Build history of the part. All positions in model axes, mm. Round coordinates to 2 decimals unless told otherwise and drop trailing zeros. Write each loop counter-clockwise with the first axis right and the second up, starting at its lowest first coordinate (ties: lowest second). Pieces come first, ordered by that corner, then holes.
from build123d import *

# Parameters (mm, degrees)
EXTRUDE_1_DEPTH     = 75
CUT_EXTRUDE_1_DEPTH = 5


with BuildPart() as part:
    # ｽｹｯﾁ1 → ﾎﾞｽ - 押し出し1 (new body)
    with BuildSketch(Plane(origin=(0, 0, 0), x_dir=(1, 0, 0), z_dir=(0, 1, 0))):
        with BuildLine():
            Line((-4, -5), (4, -5))
            ThreePointArc((4, -5), (4.707106781, -4.707106781), (5, -4))
            Line((5, -4), (5, 4))
            ThreePointArc((5, 4), (4.707106781, 4.707106781), (4, 5))
            Line((4, 5), (-4, 5))
            ThreePointArc((-4, 5), (-4.707106781, 4.707106781), (-5, 4))
            Line((-5, 4), (-5, -4))
            ThreePointArc((-5, -4), (-4.707106781, -4.707106781), (-4, -5))
        make_face()
    extrude(amount=EXTRUDE_1_DEPTH)

    # ｽｹｯﾁ2 → ｶｯﾄ - 押し出し1 (cut)
    with BuildSketch(Plane(origin=(0, 75, 0), x_dir=(1, 0, 0), z_dir=(0, 1, 0))):
        with BuildLine():
            Line((-1.6, -2.6), (1.6, -2.6))
            ThreePointArc((1.6, -2.6), (2.307106781, -2.307106781), (2.6, -1.6))
            Line((2.6, -1.6), (2.6, 1.6))
            ThreePointArc((2.6, 1.6), (2.307106781, 2.307106781), (1.6, 2.6))
            Line((1.6, 2.6), (-1.6, 2.6))
            ThreePointArc((-1.6, 2.6), (-2.307106781, 2.307106781), (-2.6, 1.6))
            Line((-2.6, 1.6), (-2.6, -1.6))
            ThreePointArc((-2.6, -1.6), (-2.307106781, -2.307106781), (-1.6, -2.6))
        make_face()
    extrude(amount=-CUT_EXTRUDE_1_DEPTH, mode=Mode.SUBTRACT)


solid = part.part
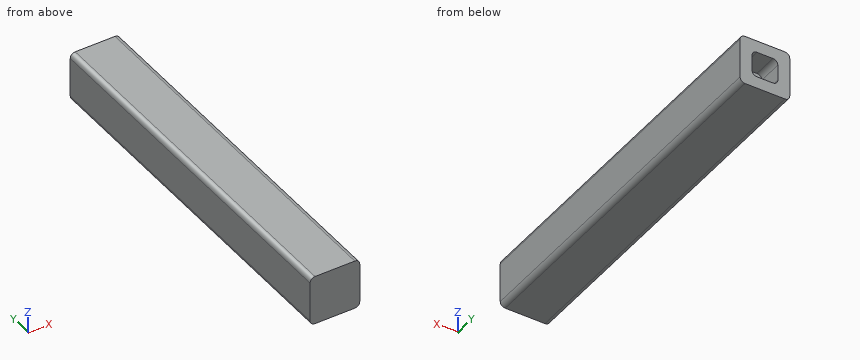
1) Wall check: L1, parallel to Y at x = 2.25, z = -0.5; L2, parallel to X at y = 43.5, z = -4.25; L3, parallel to X at y = 63, z = 4.5. Give the ranges that are in metal, low to high.
Results:
L1: y = 0 to 70
L2: x = -4.97 to 4.97
L3: x = -4.87 to 4.87
2) Slice it at A-A (x = -0.25). Write the cut outline in (y, z), plus the area to 3 significant figures.
Results:
outline: (0, -5) - (75, -5) - (75, -2.6) - (70, -2.6) - (70, 2.6) - (75, 2.6) - (75, 5) - (0, 5) - close
area: 724 mm2
3) Slice it at B-B (z = -0.25). Write the cut outline in (x, y), plus the area to 3 significant figures.
Results:
outline: (-5, 0) - (5, 0) - (5, 75) - (2.6, 75) - (2.6, 70) - (-2.6, 70) - (-2.6, 75) - (-5, 75) - close
area: 724 mm2
4) Pin check, flat tip, straight feed: pin 1 Ø2.5 at (x, z) = (1, -0.5) entering from +Y. Stop position of the tip, or through.
Results:
pin 1: stops at y = 70
